```python
from build123d import *

# Parameters (mm, degrees)
SKETCH1_R           = 75
BOSS_EXTRUDE1_DEPTH = 30
BOSS_EXTRUDE2_DEPTH = 30


with BuildPart() as part:
    # Sketch1 → Boss-Extrude1 (new body)
    with BuildSketch(Plane.XY):
        Circle(SKETCH1_R)
    extrude(amount=BOSS_EXTRUDE1_DEPTH)

    # Sketch4 → Boss-Extrude2 (add)
    with BuildSketch(Plane.XY.offset(30)):
        with BuildLine():
            Line((61.317279836, -73.033008589), (53.033008589, -53.033008589))
            ThreePointArc((53.033008589, -53.033008589), (28.701257427, -69.290964938), (0, -75))
            Line((0, -75), (8.284271247, -95))
            Line((8.284271247, -95), (61.317279836, -73.033008589))
        make_face()
        with BuildLine():
            ThreePointArc((53.033008589, 53.033008589), (69.290964938, 28.701257427), (75, 0))
            Line((75, 0), (95, 8.284271247))
            Line((95, 8.284271247), (73.033008589, 61.317279836))
            Line((73.033008589, 61.317279836), (53.033008589, 53.033008589))
        make_face()
        with BuildLine():
            Line((-73.033008589, -61.317279836), (-53.033008589, -53.033008589))
            ThreePointArc((-53.033008589, -53.033008589), (-69.290964938, -28.701257427), (-75, 0))
            Line((-75, 0), (-95, -8.284271247))
            Line((-95, -8.284271247), (-73.033008589, -61.317279836))
        make_face()
        with BuildLine():
            ThreePointArc((0, 75), (0.359885979, 74.999136542), (0.719763671, 74.996546189))
            Line((0.719763671, 74.996546189), (-6.58190731, 93.206479314))
            Line((-6.58190731, 93.206479314), (-60.476372238, 71.596314803))
            Line((-60.476372238, 71.596314803), (-53.033008589, 53.033008589))
            ThreePointArc((-53.033008589, 53.033008589), (-28.701257427, 69.290964938), (0, 75))
        make_face()
    extrude(amount=-BOSS_EXTRUDE2_DEPTH)


solid = part.part
```
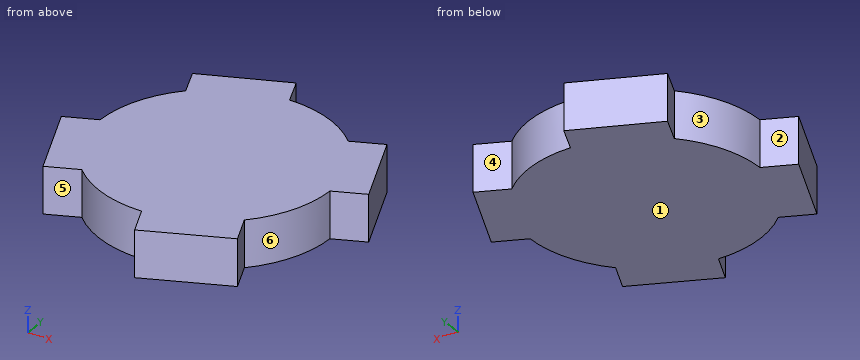
Build history of the part. All positions in model axes, mm. Face numbers are marked on the shaded views. A direction names the side the tool comes from. Coordinates: 2 decimals unless noted, no trailing zeros. Order: outer loops, then holes, each group sorted by start corner. A loop starts at its lowest first (then second) coordinate and runs counter-clockwise, first axis right, second up.
Item 1: Drop flat-ended pins along their axis: pin 1 Ø1 at (x, y) = (-76, -18.5) entering from -Z; pin 2 Ø3 at (x, z) = (-10, 15.5) entering from -Y; pin 3 Ø5 at (y, z) = (-27.5, 17.5) entering from +X; pin 4 Ø1 at (y, z) = (-35.5, 23.5) entering from -X. Give the stop position or say it passes through.
Filled in:
pin 1: stops at z = 0
pin 2: stops at y = -74.52
pin 3: stops at x = 70.71
pin 4: stops at x = -83.93
Item 2: Saw through at D-D on x = 33. List the corners of the cut face in (y, z), then the cut area to 3 significant figures.
Filled in:
outline: (-84.76, 0) - (67.35, 0) - (67.35, 30) - (-84.76, 30) - close
area: 4,560 mm2
Item 3: Mould opens along Y. For the marked faces 1, 2 and 3 say: released by +Y, released by -Y, zero draft, split by the parting line, or undercut.
Filled in:
face 1: zero draft
face 2: released by +Y
face 3: undercut
Item 4: Tool access for the marked faces 4, 5 and 6: list every direction of +Z, -Z, +X, -X, +Y, -Y with a clear straight run to the whole face (end or side of a thin tool).
Filled in:
face 4: +Z, -Z, +Y
face 5: +Z, -Z, -Y
face 6: +Z, -Z, +X
Item 5: Saw through at B-B on x = 56. List the corners of the cut face in (y, z).
Filled in:
outline: (-75.24, 0) - (-60.2, 0) - (-60.2, 30) - (-75.24, 30) - close; (-49.89, 0) - (54.26, 0) - (54.26, 30) - (-49.89, 30) - close
Item 6: Drill centre lines: L1, parallel to X at y = -59, z = 21.75; L2, parallel to X at y = -11.5, z = 17.75; L3, parallel to X at y = 48, z = 6.75. Where is each one in solid material? Low to high.
Filled in:
L1: x = -73.99 to -67.44, -46.3 to 55.5
L2: x = -93.67 to 74.11
L3: x = -57.63 to 78.55
Item 7: Saw through at A-A on z = 27. List the corners of the cut face in (x, y).
Filled in:
outline: (-95, -8.28) - (-73.03, -61.32) - (-53.03, -53.03) arc R75 ccw to (0, -75) - (8.28, -95) - (61.32, -73.03) - (53.03, -53.03) arc R75 ccw to (75, 0) - (95, 8.28) - (73.03, 61.32) - (53.03, 53.03) arc R75 ccw to (0.72, 75) - (-6.58, 93.21) - (-60.48, 71.6) - (-53.03, 53.03) arc R75 ccw to (-75, 0) - close
Item 8: Saw through at C-C on y = -82. List the corners of the cut face in (x, z), then the cut area to 3 significant figures.
Filled in:
outline: (2.9, 0) - (39.67, 0) - (39.67, 30) - (2.9, 30) - close
area: 1,100 mm2
